from build123d import *

# Parameters (mm, degrees)
SKETCH_R     = 66.350029
PAD_DEPTH    = 10
POCKET_DEPTH = 10.001


with BuildPart() as part:
    # Sketch → Pad (new body)
    with BuildSketch(Plane.XY):
        Circle(SKETCH_R)
    extrude(amount=PAD_DEPTH)

    # Sketch001 (on Face3 of Pad) → Pocket (cut, through all)
    with BuildSketch(Plane.XY.offset(10)):
        with BuildLine():
            ThreePointArc((-5, 19.364917), (0, -20), (5, 19.364917))
            Line((5, 19.364917), (5, 24.364917))
            Line((5, 24.364917), (-5, 24.364917))
            Line((-5, 24.364917), (-5, 19.364917))
        make_face()
    extrude(amount=-POCKET_DEPTH, mode=Mode.SUBTRACT)


solid = part.part
Geometry check sheet. Reference: the model listing, model coordinates, mm. A direction names the side the tool comes from. Give positions to 0.01 mm unless a question says otherwise; leave off trailing zeros. Write each loop counter-clockwise with the first axis right and the second up, starting at its lowest first coordinate (ties: lowest second). Pieces come first, ordered by that corner, then holes. Notation, with made-up numbers: (32.5, 13.25) - (41.5, 13.25) arc R22 ccw to (41.5, 49.25) - close; hole circle Ø1 at (35, 69). An arc over 180 degrees is marked (long way). Put each result on its own line as item: value.
1. Go/stop test with flat-tipped pins: pin 1 (5.5 mm diameter, centred on y = 22.5, z = 3, fed in from -X); pin 2 (6 mm diameter, centred on y = 9.5, z = 2.5, fed in from +X); pin 3 (1.5 mm diameter, centred on x = -43.5, y = -25.5, fed in from -Z); pin 4 (5 mm diameter, centred on x = 38, z = 4.5, fed in from +Y). Record where each tip stops, or that it passes through.
Ans:
pin 1: stops at x = -63.34
pin 2: stops at x = 66.03
pin 3: stops at z = 0
pin 4: stops at y = 56.05
2. Sectioned sample at C-C, the plane z = 7.25. Enter the section's corners in (x, y).
Ans:
outline: circle Ø132.7 at (0, 0); hole (-5, 19.36) arc R20 ccw (long way) to (5, 19.36) - (5, 24.36) - (-5, 24.36) - close
3. Sectioned sample at B-B, the plane y = 0. Enter the section's corners in (x, z).
Ans:
outline: (-66.35, 0) - (-20, 0) - (-20, 10) - (-66.35, 10) - close; (20, 0) - (66.35, 0) - (66.35, 10) - (20, 10) - close
4. Sectioned sample at A-A, the plane x = 0. Enter the section's corners in (y, z).
Ans:
outline: (-66.35, 0) - (-20, 0) - (-20, 10) - (-66.35, 10) - close; (24.36, 0) - (66.35, 0) - (66.35, 10) - (24.36, 10) - close
5. Set-up check for faces 4 (the flat face through (-16, -14, 10)), 5 (the flat face through (0, 24.365, 5)): record each of +Z, -Z, +X, -X, +Y, -Y from which the full face is reachable in a straight line by a thin tool's end or side.
Ans:
face 4: +Z, +X, -X, +Y, -Y
face 5: +Z, -Z
6. Draft check along X on faces 1 (the flat face through (-16, -14, 0)), 2 (the cylindrical face through (-52.653, -40.373, 4.93)), 3 (the flat face through (5, 22, 5)). Enter one of: +X half, -X half, draft (parallel to the pull), parting line (faces both ways), or undercut.
Ans:
face 1: draft
face 2: parting line
face 3: undercut
7. Thickness scan on line 1 (Y direction, x = 0, z = 7); line 2 (Y direction, x = 8.5, z = 3); line 3 (X direction, y = 10, z = 7.5). Record the ranges inside material, lowest first.
Ans:
line 1: y = -66.35 to -20, 24.36 to 66.35
line 2: y = -65.8 to -18.1, 18.1 to 65.8
line 3: x = -65.59 to -17.32, 17.32 to 65.59
8. Sectioned sample at D-D, the plane x = -46. Enter the section's corners in (y, z), plus the area to 3 significant figures.
Ans:
outline: (-47.82, 0) - (47.82, 0) - (47.82, 10) - (-47.82, 10) - close
area: 956 mm²
